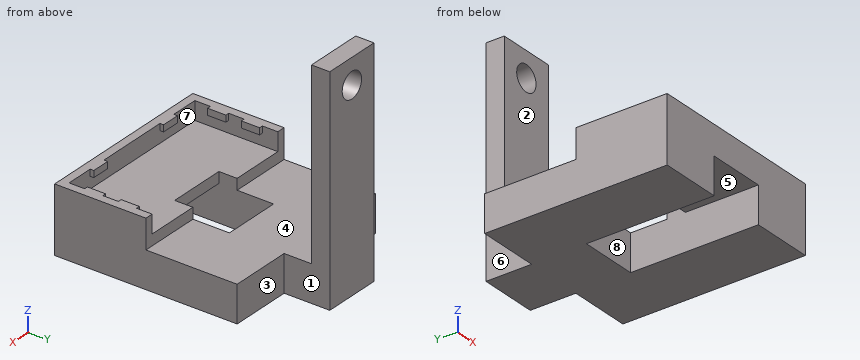
Autodesk Inventor part; units mm, degrees
ref_plane "YZ Plane" through (0, 0, 0) normal (1, 0, 0) x (0, 1, 0)
ref_plane "XZ Plane" through (0, 0, 0) normal (0, 1, 0) x (-1, 0, 0)
ref_plane "XY Plane" through (0, 0, 0) normal (0, 0, 1) x (1, 0, 0)
sketch "Sketch1" plane through (0, 0, 0) normal (0, 0, 1) x (1, 0, 0)
  line L0 (-25, 12.5) -> (25, 12.5)
  line L1 (25, 12.5) -> (25, -12.5)
  line L2 (25, -12.5) -> (-25, -12.5)
  line L3 (-25, -12.5) -> (-25, 12.5)
  line L4 (-25, 12.5) -> (25, -12.5) construction
  line L5 (25, 12.5) -> (-25, -12.5) construction
  line L6 (-25, 12.5) -> (25, 12.5) construction
  point P0 (0, 0)
  dimension "d0" = 50
  dimension "d1" = 0
  dimension "d2" = 25
extrude "Extrusion1" add sketch "Sketch1" along normal blind 3
sketch "Sketch2" plane through (0, 0, 3) normal (0, 0, 1) x (1, 0, 0)
  line L0 (-22.75, -10.25) -> (22.75, -10.25)
  line L1 (22.75, -10.25) -> (22.75, 10.25)
  line L2 (22.75, 10.25) -> (-22.75, 10.25)
  line L3 (-22.75, 10.25) -> (-22.75, -10.25)
  line L4 (-22.75, -10.25) -> (22.75, 10.25) construction
  line L5 (22.75, -10.25) -> (-22.75, 10.25) construction
  line L6 (-22.75, -10.25) -> (22.75, -10.25) construction
  line L7 (25, 12.5) -> (-25, 12.5)
  line L8 (-25, -12.5) -> (25, -12.5)
  line L9 (25, 12.5) -> (25, -12.5)
  line L10 (25, -12.5) -> (-25, -12.5)
  line L11 (-25, -12.5) -> (-25, 12.5)
  line L12 (-22.75, 10.25) -> (-22.75, 12.5)
  line L13 (22.75, 10.25) -> (22.75, 12.5)
  line L14 (-25, 12.5) -> (-22.75, 12.5)
  line L15 (22.75, 12.5) -> (25, 12.5)
  point P0 (0, 0)
  dimension "d5" = 45.5
  dimension "d6" = 0
  dimension "d7" = 20.5
extrude "Extrusion2" add sketch "Sketch2" along normal blind 5 contours L0 L1 L13 L7 L9 L8 L11 L12 L3
sketch "Sketch3" plane through (-22.75, -10.25, 3) normal (1, 0, 0) x (0, 0, -1)
  line L0 (-5, 0) -> (-5, 22.75)
  line L1 (-3.2, 18.5) -> (-5, 18.5)
  line L2 (-5, 18.5) -> (-5, 13.5)
  line L3 (-5, 13.5) -> (-3.2, 13.5)
  line L4 (-3.2, 13.5) -> (-3.2, 18.5)
  line L5 (-5, 4.25) -> (-3.2, 4.25)
  line L6 (-3.2, 4.25) -> (-3.2, 9.25)
  line L7 (-3.2, 9.25) -> (-5, 9.25)
  line L8 (-5, 9.25) -> (-5, 4.25)
  point P0 (3, 10.25)
  point P1 (-5, 9.25)
  point P2 (-5, 4.25)
  dimension "d10" = 5
  dimension "d11" = 5
  dimension "d28" = 1.8
extrude "Extrusion3" add sketch "Sketch3" along normal blind 1
sketch "Sketch4" plane through (22.75, -10.25, 3) normal (-1, 0, 0) x (0, 0, 1)
  line L0 (5, 18.5) -> (5, 13.5)
  line L1 (3.2, 13.5) -> (3.2, 18.5)
  line L2 (5, 18.5) -> (3.2, 18.5)
  line L3 (3.2, 18.5) -> (3.2, 13.5)
  line L4 (3.2, 13.5) -> (5, 13.5)
  line L5 (5, 13.5) -> (5, 18.5)
  line L6 (5, 9.25) -> (5, 13.5)
  line L7 (3.2, 9.25) -> (3.2, 4.25)
  line L8 (5, 9.25) -> (3.2, 9.25)
  line L9 (3.2, 9.25) -> (3.2, 4.25)
  line L10 (3.2, 4.25) -> (5, 4.25)
  line L11 (5, 4.25) -> (5, 9.25)
  point P0 (-3, 10.25)
extrude "Extrusion4" add sketch "Sketch4" along normal blind 1
sketch "Sketch5" plane through (-22.75, -10.25, 3) normal (0, 1, 0) x (1, 0, 0)
  line L0 (45.5, -5) -> (0, -5)
  line L1 (7.625, -5) -> (12.625, -5)
  line L2 (12.625, -5) -> (12.625, -3.2)
  line L3 (12.625, -3.2) -> (7.625, -3.2)
  line L4 (7.625, -3.2) -> (7.625, -5)
  line L5 (32.875, -5) -> (37.875, -5)
  line L6 (37.875, -5) -> (37.875, -3.2)
  line L7 (37.875, -3.2) -> (32.875, -3.2)
  line L8 (32.875, -3.2) -> (32.875, -5)
  point P0 (22.75, 3)
  dimension "d31" = 5
  dimension "d32" = 1.8
  dimension "d33" = 5
  dimension "d34" = 1.8
extrude "Extrusion5" add sketch "Sketch5" along normal blind 1
sketch "Sketch6" plane through (0, 0, 0) normal (0, 0, -1) x (-1, 0, 0)
  line L0 (25, -12.5) -> (-25, -12.5)
  line L1 (-8, -12.5) -> (-25, -12.5)
  line L2 (-25, -12.5) -> (-25, 37.5)
  line L3 (-25, 37.5) -> (-8, 37.5)
  line L4 (-8, 37.5) -> (-8, -12.5)
  line L5 (8, -12.5) -> (25, -12.5)
  line L6 (25, -12.5) -> (25, 37.5)
  line L7 (25, 37.5) -> (8, 37.5)
  line L8 (8, 37.5) -> (8, -12.5)
  line L9 (-8, 50) -> (-8, 22.5)
  line L10 (-8, 22.5) -> (8, 22.5)
  line L11 (-8, 50) -> (8, 50)
  line L12 (-8, 50) -> (8, 50) construction
  line L13 (8, 50) -> (8, 37.5)
  point P0 (0, 0)
  point P1 (-25, -12.5)
  point P2 (25, -12.5)
  point P3 (8, 50)
  dimension "d41" = 17
  dimension "d42" = 50
  dimension "d43" = 17
  dimension "d44" = 50
  dimension "d47" = 16
  dimension "d49" = 0
extrude "Extrusion6" add sketch "Sketch6" along normal blind 10 contours L0 L8 L7 L6 | L0 L2 L3 L4 | L10 L4 L9 L11 L13 L8
sketch "Sketch7" plane through (0, 0, 3) normal (0, 0, 1) x (1, 0, 0)
  line L0 (22.75, 12.5) -> (-22.75, 12.5)
  line L1 (-8, 12.5) -> (8, 12.5)
  line L2 (8, 12.5) -> (8, 7.5)
  line L3 (8, 7.5) -> (-8, 7.5)
  line L4 (-8, 7.5) -> (-8, 12.5)
  point P0 (0, 0)
  dimension "d35" = 16
  dimension "d36" = 5
extrude "Extrusion7" cut sketch "Sketch7" against normal through all
sketch "Sketch18" plane through (-8, 50, 0) normal (0, 1, 0) x (1, 0, 0)
  line L0 (0, 0) -> (16, 0)
  line L1 (0, 0) -> (16, 0)
  line L2 (16, 0) -> (16, -50)
  line L3 (16, -50) -> (0, -50)
  line L4 (0, -50) -> (0, 0)
  line L5 (16, 0) -> (16, 10)
  circle A0 centre (8, -43) radius 3.5
  point P0 (8, 0)
  point P1 (8, 0)
  dimension "d86" = 50
  dimension "d87" = 7
  dimension "d88" = 7
extrude "Extrusion15" add sketch "Sketch18" against normal blind 5
properties part number "sensor mount"
Design review of the part built by this model. Coordinates are the model's own, in mm. Face numbers are marked on the shaded views. A direction names the side the tool comes from. Coordinates: 2 decimals unless noted, no trailing zeros. Order: outer loops, then holes, each group sorted by start corner. A loop starts at its lowest first (then second) coordinate and runs counter-clockwise, first axis right, second up.
1) Take a section at B-B, the plane x = -4.5. Give the boundary of the cut face in (y, z), and give its area (3 significant figures).
2) Take a section at A-A, the plane z = 43. Give the boundary of the cut face in (x, y).
3) Clearance check with flat-ended pins moving along their axes: pin 1 (25 mm diameter, centred on x = -8, y = 4.5, fed in from +Z); pin 2 (3 mm diameter, centred on x = -16.5, z = -5.5, fed in from +Y); pin 3 (6 mm diameter, centred on y = 45, z = 11.5, fed in from -X). State where each tip first meets the part, or that it passes through.
4) Take a section at C-C, the plane y = 21.5. Give the boundary of the cut face in (x, z).
5) Wall thickness on line 1 along Z through (x, y) = (0, 46.2); line 2 along X through (y, z) = (47.4, 43); line 3 along Y through (x, z) = (-6, 6.5): over which ranges is each line inside the solid? List them lowest first.
6) Mouldability with a two-part tool opening along Y and no side actions: class the marked faces 1, 2 and 3 as +Y half, -Y half, draft (parallel to the pull), parting line (faces both ways), or undercut.
7) Take a section at D-D, the plane x = 0.5. Give the boundary of the cut face in (y, z).
8) For the marked faces 4, 5, 6, 7 and 8, list the 3-axis set-ups (+Z, -Z, +X, -X, +Y, -Y) from which the entire face can be reached by the end or side of a thin tool; tool diameter is ignored.
Returned:
1. outline: (-12.5, 0) - (7.5, 0) - (7.5, 3) - (-10.25, 3) - (-10.25, 8) - (-12.5, 8) - close; (22.5, -10) - (50, -10) - (50, 50) - (45, 50) - (45, 0) - (22.5, 0) - close
1. area: 596 mm2
2. outline: (-8, 45) - (-3.5, 45) - (-3.5, 50) - (-8, 50) - close; (3.5, 45) - (8, 45) - (8, 50) - (3.5, 50) - close
3. pin 1: stops at z = 3
3. pin 2: stops at y = 37.5
3. pin 3: stops at x = -8
4. outline: (-25, -10) - (-8, -10) - (-8, 0) - (-25, 0) - close; (8, -10) - (25, -10) - (25, 0) - (8, 0) - close
5. line 1: z = -10 to 39.5, 46.5 to 50
5. line 2: x = -8 to -3.5, 3.5 to 8
5. line 3: y = -12.5 to -10.25, 45 to 50
6. face 1: draft
6. face 2: undercut
6. face 3: +Y half
7. outline: (-12.5, 0) - (7.5, 0) - (7.5, 3) - (-10.25, 3) - (-10.25, 8) - (-12.5, 8) - close; (22.5, -10) - (50, -10) - (50, 39.54) - (45, 39.54) - (45, 0) - (22.5, 0) - close; (45, 46.46) - (50, 46.46) - (50, 50) - (45, 50) - close
8. face 4: +Z, +X, -X
8. face 5: -Z, -Y
8. face 6: +Z, -Z, -X, +Y
8. face 7: none
8. face 8: +Z, -Z, -Y
